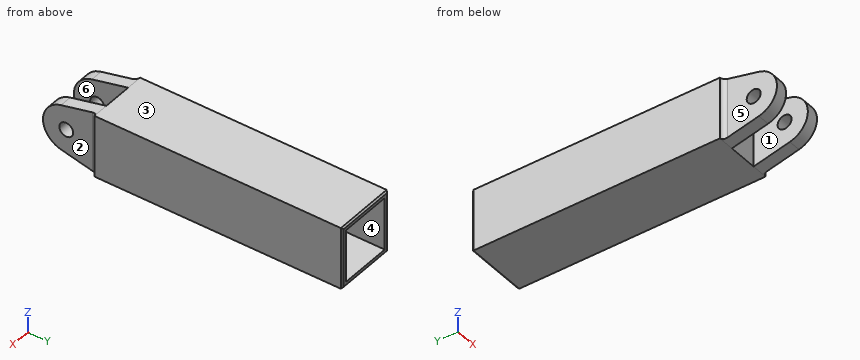
from build123d import *

# Parameters (mm, degrees)
F0_W         = 160
F0_H         = 40
F1_DEPTH     = 20
F2_W         = 34
F2_H         = 34
F3_DEPTH     = 25
F4_R         = 4.5
F5_DEPTH     = 17.5
F7_DEPTH     = 25
F8_T4_DEPTH  = 54.7901994578
F8_T10_DEPTH = 54.7901994578
F9_SIZE      = 1


# Not quite as in the source:
# - a fillet or chamfer that OpenCascade refuses, or shapes differently, is made with other operations: its cross-section is extruded or revolved along the edge and cut away or added


with BuildPart() as f1:
    # F0 (on Right) → F1 (new body, symmetric)
    with BuildSketch(Plane.YZ):
        Rectangle(F0_W, F0_H)
    extrude(amount=F1_DEPTH, both=True)

    # F2 (on face) → F3 (cut)
    with BuildSketch(Plane(origin=(0, 80, 0), x_dir=(-1, 0, 0), z_dir=(0, 1, 0))):
        Rectangle(F2_W, F2_H)
    extrude(amount=-F3_DEPTH, mode=Mode.SUBTRACT)

    # F4 (on Right) → F5 (join, symmetric)
    with BuildSketch(Plane.YZ):
        with BuildLine():
            Line((-80, 20), (-103.3671841062, 14.6171841062))
            ThreePointArc((-103.3671841062, 14.6171841062), (-115, 0), (-103.3671841062, -14.6171841062))
            Line((-103.3671841062, -14.6171841062), (-80, -20))
            Line((-80, -20), (-80, 0))
            Line((-80, 0), (-80, 20))
        make_face()
        with Locations((-100, 0)):
            Circle(F4_R, mode=Mode.SUBTRACT)
    extrude(amount=F5_DEPTH, both=True)

    # F6 (on Top) → F7 (cut, symmetric)
    with BuildSketch(Plane.XY):
        Polygon((-9.5, -115), (0, -115), (9.5, -115), (9.5, -80), (-9.5, -80), align=None)
    extrude(amount=F7_DEPTH, both=True, mode=Mode.SUBTRACT)

    # F8: fillet of radius 3 on 2 edges, made by hand


with BuildPart() as f8_tool2:
    # F8_s3 → F8_t4 (new body)
    with BuildSketch(Plane.XY.offset(-27.3950997289)):
        with BuildLine():
            ThreePointArc((-17.5, -82.9580398916), (-18.2087121525, -81.0215482184), (-20, -80))
            Line((-20, -80), (-17.5, -80))
            Line((-17.5, -80), (-17.5, -82.9580398916))
        make_face()
    extrude(amount=F8_T4_DEPTH)

    split(bisect_by=Plane(origin=(0, -8.4062635752, 36.4921841062), x_dir=(1, 0, 0), z_dir=(0, 0.2244789404, -0.9744789404)), keep=Keep.TOP)

    split(bisect_by=Plane(origin=(0, -8.4062635752, -36.4921841062), x_dir=(1, 0, 0), z_dir=(0, 0.2244789404, 0.9744789404)), keep=Keep.TOP)


with BuildPart() as f1_1:
    add(f1.part)

    # F8_t1: union F8_tool2
    add(f8_tool2.part)


with BuildPart() as f8_tool8:
    # F8_s9 → F8_t10 (new body)
    with BuildSketch(Plane.XY.offset(27.3950997289)):
        with BuildLine():
            ThreePointArc((20, -80), (18.2087121525, -81.0215482184), (17.5, -82.9580398916))
            Line((17.5, -82.9580398916), (17.5, -80))
            Line((17.5, -80), (20, -80))
        make_face()
    extrude(amount=-F8_T10_DEPTH)

    split(bisect_by=Plane(origin=(0, -8.4062635752, -36.4921841062), x_dir=(1, 0, 0), z_dir=(0, 0.2244789404, 0.9744789404)), keep=Keep.TOP)

    split(bisect_by=Plane(origin=(0, -8.4062635752, 36.4921841062), x_dir=(1, 0, 0), z_dir=(0, 0.2244789404, -0.9744789404)), keep=Keep.TOP)


with BuildPart() as f1_2:
    add(f1_1.part)

    # F8_t7: union F8_tool8
    add(f8_tool8.part)

    # F9
    f9_edges = [f1_2.edges().sort_by_distance(p)[0] for p in [
        (0, 80, 20),
        (-20, 80, 0),
        (0, 80, -20),
        (20, 80, 0),
    ]]
    chamfer(f9_edges, length=F9_SIZE)


solid = f1_2.part
Verification items for the finished model (mm, model axes). Face numbers are marked on the shaded views. A direction names the side the tool comes from. Coordinates: 2 decimals unless noted, no trailing zeros. Write each loop counter-clockwise with the first axis right and the second up, starting at its lowest first coordinate (ties: lowest second). Pieces come first, ordered by that corner, then holes. Notation, with made-up numbers: M 17,77 L 75,77 A16 ccw 75,101 Z; hole C 7.25,23 d4. An arc over 180 degrees is marked long. Use CSV: the item, a comma, the result in double quotes.
Q1. Section check B-B, the plane y = -100. Enter the section's corners in (x, z).
Computed values:
outline,"M -17.5,-15.39 L -9.5,-15.39 L -9.5,-4.5 L -17.5,-4.5 Z; M -17.5,4.5 L -9.5,4.5 L -9.5,15.39 L -17.5,15.39 Z; M 9.5,-15.39 L 17.5,-15.39 L 17.5,-4.5 L 9.5,-4.5 Z; M 9.5,4.5 L 17.5,4.5 L 17.5,15.39 L 9.5,15.39 Z"
Q2. Mould release check, pull along X, two halves, no side actions. Record for the marked faces 1, 2 and 3: pulls with the +X half, pulls with the -X half, needs draft (parallel to the pull), parting line crosses it, or undercut.
Computed values:
face 1,"undercut"
face 2,"pulls with the +X half"
face 3,"needs draft"
Q3. Set-up check for the marked faces 4, 5 and 6: record each of +Z, -Z, +X, -X, +Y, -Y from which the full face is reachable in a straight line by a thin tool's end or side.
Computed values:
face 4,"+Y"
face 5,"+Z, -Z, -X, -Y"
face 6,"+Z, -Z, -Y"
Q4. Section check A-A, the plane x = -0.5. Enter the section's corners in (y, z), and give its area (3 significant figures).
Computed values:
outline,"M -80,-20 L 79,-20 L 80,-19 L 80,-17 L 55,-17 L 55,17 L 80,17 L 80,19 L 79,20 L -80,20 Z"
area,"5,550 mm²"
Q5. Go/stop test with flat-tipped pins: P1, Ø3, axis at x = 11, z = -3.5, coming from the -Y side; P2, Ø10, axis at x = 8.5, z = 0, coming from the +Y side; P3, Ø16, axis at y = -92, z = 1.5, coming from the -X side; P4, Ø15, axis at x = -3, z = -2.5, coming from the -Y side. Record where each tip stops, or that it passes through.
Computed values:
P1,"y = -114.87"
P2,"y = 55"
P3,"x = -17.5"
P4,"y = -115"
Q6. Thickness scan on line 1 along Y through (x, z) = (-12.25, 0); line 2 along X through (y, z) = (59, -9); line 3 along Y through (x, z) = (4.5, 16.5). Record the ranges inside material, lowest first. Write a range as [from, to].
Computed values:
line 1,"[-115, -104.5], [-95.5, 55]"
line 2,"[-20, -17], [17, 20]"
line 3,"[-80, 55]"
